from build123d import *

# Parameters (mm, degrees)
SKETCH_1_W             = 96.558139534
SKETCH_1_H             = 40
EXTRUDE_1_DEPTH        = 51
SKETCH_2_W             = 96.558139534
SKETCH_2_H             = 20
EXTRUDE_2_DEPTH        = 20
SKETCH_4_W             = 38.279069767
SKETCH_4_H             = 17
CUT_EXTRUDE_1_DEPTH    = 17
CUT_EXTRUDE_2_DEPTH    = 112.015648944
HOLE_WIZARD_M4_1_D     = 3.8
HOLE_WIZARD_M4_1_DEPTH = 10.1
HOLE_WIZARD_M4_1_TIP   = 1.141635176
SKETCH_9_W             = 25.779069767
SKETCH_9_H             = 40
CUT_EXTRUDE_3_DEPTH    = 51
EXTRUDE_START          = -45
EXTRUDE_4_DEPTH        = 45
SKETCH_11_W            = 45
SKETCH_11_H            = 20
CUT_EXTRUDE_4_DEPTH    = 0.8


with BuildPart() as part:
    # 스케치1 → 보스-돌출1 (new body)
    with BuildSketch(Plane.XY):
        Rectangle(SKETCH_1_W, SKETCH_1_H)
    extrude(amount=EXTRUDE_1_DEPTH)

    # 스케치2 → 보스-돌출2 (add)
    with BuildSketch(Plane(origin=(0, 0, 0), x_dir=(-1, 0, 0), z_dir=(0, 0, -1))):
        with Locations((0, 10)):
            Rectangle(SKETCH_2_W, SKETCH_2_H)
    extrude(amount=EXTRUDE_2_DEPTH)

    # 스케치4 → 컷-돌출1 (cut)
    with BuildSketch(Plane(origin=(0, 20, 0), x_dir=(1, 0, 0), z_dir=(0, 1, 0))):
        with Locations((-24.139534884, 11.5)):
            Rectangle(SKETCH_4_W, SKETCH_4_H)
        with Locations((24.139534884, 11.5)):
            Rectangle(SKETCH_4_W, SKETCH_4_H)
    extrude(amount=-CUT_EXTRUDE_1_DEPTH, mode=Mode.SUBTRACT)

    # 스케치6 → 컷-돌출2 (cut, through all)
    with BuildSketch(Plane(origin=(48.279069767, 0, 0), x_dir=(0, 0, -1), z_dir=(1, 0, 0))):
        Polygon((3, 20), (20, 20), (20, 3), align=None)
    extrude(amount=-CUT_EXTRUDE_2_DEPTH, mode=Mode.SUBTRACT)

    # M4 나사 구멍1
    with Locations(Plane(origin=(0, 3, 0), x_dir=(1, 0, 0), z_dir=(0, 1, 0))):
        with Locations((-33.279069767, 10), (-15, 10), (15, 10), (33.279069767, 10)):
            Hole(HOLE_WIZARD_M4_1_D / 2, depth=HOLE_WIZARD_M4_1_DEPTH)
            with Locations((0, 0, -(HOLE_WIZARD_M4_1_DEPTH + HOLE_WIZARD_M4_1_TIP / 2))):  # 118° drill point
                Cone(0, HOLE_WIZARD_M4_1_D / 2, HOLE_WIZARD_M4_1_TIP, mode=Mode.SUBTRACT)

    # 스케치9 → 컷-돌출3 (cut)
    with BuildSketch(Plane.XY.offset(51)):
        with Locations((-35.389534884, 0)):
            Rectangle(SKETCH_9_W, SKETCH_9_H)
        with Locations((35.389534884, 0)):
            Rectangle(SKETCH_9_W, SKETCH_9_H)
    extrude(amount=-CUT_EXTRUDE_3_DEPTH, mode=Mode.SUBTRACT)

    # 스케치10 → 보스-돌출4 (add)
    with BuildSketch(Plane.ZY.offset(22.5).offset(EXTRUDE_START)):
        Polygon((51, 20), (51, 41), (0, 20), align=None)
    extrude(amount=EXTRUDE_4_DEPTH)

    # 스케치11 → 컷-돌출4 (cut)
    with BuildSketch(Plane(origin=(0, 0, 0), x_dir=(-1, 0, 0), z_dir=(0, 0, -1))):
        with Locations((0, -10)):
            Rectangle(SKETCH_11_W, SKETCH_11_H)
    extrude(amount=-CUT_EXTRUDE_4_DEPTH, mode=Mode.SUBTRACT)


solid = part.part
Can you work these out from the model? Positions are in its coordinate system, mm. A direction names the side the tool comes from. Give positions to 0.01 mm unless a question says otherwise; leave off trailing zeros. Order: outer loops, then holes, each group sorted by start corner. A loop starts at its lowest first (then second) coordinate and runs counter-clockwise, first axis right, second up. Notation, with made-up numbers: M 9.5,16.5 L 27.5,16.5 A22 ccw 27.5,39.5 Z; hole C -26.75,33 d4. An arc over 180 degrees is marked long. Use one line per item in the form item = value.
Item 1: If I drill on line 1 along X through (y, z) = (2.2, -10); line 2 along Z through (x, y) = (-15, 1.75); line 3 along Y through (x, z) = (26.5, -14), over which ranges is the centre line in solid material (lowest first)? Write a range as [from, to].
Values follow:
line_1 = [-48.28, -35.18], [-31.38, -16.9], [-13.1, 13.1], [16.9, 31.38], [35.18, 48.28]
line_2 = [-20, -11.9], [-8.1, 51]
line_3 = [0, 3]
Item 2: Will these pins go through, and if not, where does the flat tip stop? pin 1 Ø6 at (x, y) = (1.5, -12.5) entering from -Z; pin 2 Ø5 at (y, z) = (13, -14) entering from +X; pin 3 Ø10 at (x, z) = (-5.5, 41.5) entering from +Y; pin 4 Ø23 at (x, z) = (-9, -8) entering from -Y.
Values follow:
pin_1 = 0.8
pin_2 = through
pin_3 = 39.15
pin_4 = -20
Item 3: If we section it at A-A, the plane z = -10: Write out the boundary of the cut face in (x, y), and give its area (3 significant figures).
Values follow:
outline = M -48.28,0 L -35.18,0 L -35.18,3 L -43.28,3 L -43.28,13 L -48.28,13 Z; M -31.38,0 L -16.9,0 L -16.9,3 L -31.38,3 Z; M -13.1,0 L 13.1,0 L 13.1,3 L 5,3 L 5,13 L -5,13 L -5,3 L -13.1,3 Z; M 16.9,0 L 31.38,0 L 31.38,3 L 16.9,3 Z; M 35.18,0 L 48.28,0 L 48.28,13 L 43.28,13 L 43.28,3 L 35.18,3 Z
area = 444 mm^2
Item 4: If we section it at C-C, the plane y = 8.5: Write out the boundary of the cut face in (x, z).
Values follow:
outline = M -48.28,-14.5 L -43.28,-14.5 L -43.28,-3 L -5,-3 L -5,-14.5 L 5,-14.5 L 5,-3 L 43.28,-3 L 43.28,-14.5 L 48.28,-14.5 L 48.28,0 L 22.5,0 L 22.5,51 L -22.5,51 L -22.5,0 L -48.28,0 Z
Item 5: If we section it at D-D, the plane x = 3.5: Write out the boundary of the cut face in (y, z), and give its area (4 significant figures).
Values follow:
outline = M -20,0.8 L 0,0.8 L 0,-20 L 3,-20 L 20,-3 L 20,0 L 41,51 L -20,51 Z
area = 2,815 mm^2
Item 6: For faces 1 (the flat face through (-22.5, 4, 25)), 2 (the flat face through (22.5, 4, 25)), 3 (the flat face through (-24, 12, -3)), 4 (the flat face through (1, 20, -1)), which set-ups out of +Z, -Z, +X, -X, +Y, -Y let a thin tool reach every point of the face, with its end or its side?
Values follow:
face_1 = +Z, -X, +Y, -Y
face_2 = +Z, +X, +Y, -Y
face_3 = -Z, +Y
face_4 = -Z, +X, -X, +Y
Item 7: If we section it at B-B, the plane x = 15: Write out the boundary of the cut face in (y, z), and give its area (3 significant figures).
Values follow:
outline = M -20,0.8 L 0,0.8 L 0,-8.1 L 3,-8.1 L 3,-3 L 20,-3 L 20,0 L 41,51 L -20,51 Z; M 0,-20 L 3,-20 L 3,-11.9 L 0,-11.9 Z
area = 2,660 mm^2
Item 8: Thinking about a two-plate mould opening in X: for faces 5 (the flat face through (48.279, 8, -8)), 6 (the flat face through (24, 12, -3)), 7 (the flat face through (0, 11, -12)), 8 (the flat face through (-48.279, 8, -8)), which applies, pulls with the +X half, pulls with the -X half, needs draft (parallel to the pull), parting line crosses it, or undercut?
Values follow:
face_5 = pulls with the +X half
face_6 = undercut
face_7 = needs draft
face_8 = pulls with the -X half
